Build history of the part. All positions in model axes, mm. A direction names the side the tool comes from. Give positions to 0.01 mm unless a question says otherwise; leave off trailing zeros. Order: outer loops, then holes, each group sorted by start corner. A loop starts at its lowest first (then second) coordinate and runs counter-clockwise, first axis right, second up. Notation, with made-up numbers: (88, 68) - (142, 68) arc R12 ccw to (142, 86) - close; hole circle Ø2 at (78, -17.5). An arc over 180 degrees is marked (long way). Use a Markdown table: item, result.
from build123d import *

# Parameters (mm, degrees)
SKETCH001_R         = 1
PAD001_DEPTH        = 6
CYLINDER003_R       = 0.5
CYLINDER003_DEPTH   = 3
LINEARPATTERN_COUNT = 3
LINEARPATTERN_PITCH = 5.1


with BuildPart() as part:
    # Sketch001 → Pad001 (new body)
    with BuildSketch(Plane.XY):
        Polygon((6.4, 3.15), (6.4, -3.15), (4.3, -3.15), (4.3, -3.55), (1.9, -3.55), (1.9, -3.15), (-1.9, -3.15), (-1.9, -3.55), (-4.3, -3.55), (-4.3, -3.15), (-6.4, -3.15), (-6.4, 3.15), (-5.4, 3.15), (-5.4, 3.743355), (6.999118, 7.65), (7.119322, 7.268489), (-5, 3.45), (-5, 3.15), align=None)
        with Locations((3.25, -2.15)):
            Circle(SKETCH001_R, mode=Mode.SUBTRACT)
        with BuildLine():
            ThreePointArc((-3.708258, -1.15), (-4.35, -2.15), (-3.708258, -3.15))
            Line((-2.791742, -3.15), (-3.708258, -3.15))
            ThreePointArc((-2.791742, -3.15), (-2.15, -2.15), (-2.791742, -1.15))
            Line((-3.708258, -1.15), (-2.791742, -1.15))
        make_face(mode=Mode.SUBTRACT)
    extrude(amount=PAD001_DEPTH)

    # Cylinder003 → Cylinder003 (join)
    with BuildSketch(Plane(origin=(-5.1, -3, 3), x_dir=(1, 0, 0), z_dir=(0, -1, 0))):
        Circle(CYLINDER003_R)
    cylinder003 = extrude(amount=CYLINDER003_DEPTH)

    # LinearPattern: Cylinder003 ×3
    with Locations(*[(i * LINEARPATTERN_PITCH, 0, 0) for i in range(1, LINEARPATTERN_COUNT)]):
        add(cylinder003)


solid = part.part
1) Slice it at D-D (x = -3). Write the cut outline in (y, z).
Computed:
| item | result |
|---|---|
| outline | (-3.55, 0) - (-3.15, 0) - (-3.15, 6) - (-3.55, 6) - close; (-1.15, 0) - (3.15, 0) - (3.15, 6) - (-1.15, 6) - close; (4.08, 0) - (4.5, 0) - (4.5, 6) - (4.08, 6) - close |
2) Pin check, flat tips, straight feed: P1, Ø2, axis at y = 1, z = 1.5, coming from the +X side; P2, Ø2, axis at x = 5, z = 4, coming from the +Y side; P3, Ø0.7, axis at x = -3, z = 2.5, coming from the -Y side. Stop position of each tip, or through.
Computed:
| item | result |
|---|---|
| P1 | stops at x = 6.4 |
| P2 | stops at y = 7.34 |
| P3 | stops at y = -3.55 |
3) Slice it at B-B (z = 3.8). Write the cut outline in (x, y), and give its area (3 significant figures).
Computed:
| item | result |
|---|---|
| outline | (-6.4, -3.15) - (-4.3, -3.15) - (-4.3, -3.55) - (-1.9, -3.55) - (-1.9, -3.15) - (1.9, -3.15) - (1.9, -3.55) - (4.3, -3.55) - (4.3, -3.15) - (6.4, -3.15) - (6.4, 3.15) - (-5, 3.15) - (-5, 3.45) - (7.12, 7.27) - (7, 7.65) - (-5.4, 3.74) - (-5.4, 3.15) - (-6.4, 3.15) - close; hole (-3.71, -3.15) - (-2.79, -3.15) arc R1.1 ccw to (-2.79, -1.15) - (-3.71, -1.15) arc R1.1 ccw to start; hole circle Ø2 at (3.25, -2.15) |
| area | 81.1 mm² |
4) Tool access for faces 1 (the cylindrical face through (-0.065, -4.555, 3.496)), 2 (the flat face through (6.4, 0, 3)), 3 (the flat face through (-6, 3.15, 3)), 4 (the flat face through (1, 3.15, 3)), 5 (the cylindrical face through (-4.35, -2.13, 2.96)): list every direction of +Z, -Z, +X, -X, +Y, -Y with a clear straight run to the whole face (end or side of a thin tool).
Computed:
| item | result |
|---|---|
| face 1 | -Y |
| face 2 | +Z, -Z, +X, -Y |
| face 3 | +Z, -Z, -X, +Y |
| face 4 | +Z, -Z, +X |
| face 5 | +Z, -Z |
5) Two-plate mould, pull along Y, no slides. Class faces 6 (the flat face through (-3, -1.15, 3)), 7 (the cylindrical face through (5.577, -4.555, 3.15)), 8 (the flat face through (6, -3.15, 3)): +Y half, -Y half, draft (parallel to the pull), parting line (faces both ways), or undercut.
Computed:
| item | result |
|---|---|
| face 6 | undercut |
| face 7 | draft |
| face 8 | -Y half |
6) Wall check: line 1 (X direction, y = -3, z = 4.15); line 2 (Y direction, x = 2.5, z = 2.3); line 3 (Y direction, x = -2.5, z = 3.45). Give the ranges that are in metal, low to high. Write a range as from..to.
Computed:
| item | result |
|---|---|
| line 1 | x = -6.4..-3.95, -2.55..2.72, 3.78..6.4 |
| line 2 | y = -3.55..-2.81, -1.49..3.15, 5.81..6.23 |
| line 3 | y = -3.55..-2.95, -1.35..3.15, 4.24..4.66 |
7) Slice it at C-C (x = 0). Write the cut outline in (y, z), and give its area (3 significant figures).
Computed:
| item | result |
|---|---|
| outline | (-6, 2.5) - (-3.15, 2.5) - (-3.15, 0) - (3.15, 0) - (3.15, 6) - (-3.15, 6) - (-3.15, 3.5) - (-6, 3.5) - close; (5.03, 0) - (5.44, 0) - (5.44, 6) - (5.03, 6) - close |
| area | 43.2 mm² |
8) Slice it at A-A (y = -2.15). Write the cut outline in (x, z).
Computed:
| item | result |
|---|---|
| outline | (-6.4, 0) - (-4.35, 0) - (-4.35, 6) - (-6.4, 6) - close; (-2.15, 0) - (2.25, 0) - (2.25, 6) - (-2.15, 6) - close; (4.25, 0) - (6.4, 0) - (6.4, 6) - (4.25, 6) - close |
